```python
from build123d import *

# Parameters (mm, degrees)
SKETCH_1_R          = 3
EXTRUDE_1_DEPTH     = 4
SKETCH_2_W          = 102
SKETCH_2_H          = 85
EXTRUDE_2_DEPTH     = 50
SKETCH_4_W          = 96
SKETCH_4_H          = 79
CUT_EXTRUDE_3_DEPTH = 50
FILLET_1_R          = 4
CUT_EXTRUDE_4_REACH = 124.172
SKETCH_5_R          = 10


with BuildPart() as part:
    # 草图1 → 凸台-拉伸1 (new body)
    with BuildSketch(Plane(origin=(0, 0, 0), x_dir=(1, 0, 0), z_dir=(0, 1, 0))):
        Polygon((51, -42.5), (51, 42.5), (32.560911085, 54.5), (-32.560911085, 54.5), (-51, 42.5), (-51, -42.5), (-32.560911085, -54.5), (32.560911085, -54.5), align=None)
        with Locations(Location((-24, 48.5, 0), (0, 0, 270))):
            Circle(SKETCH_1_R, mode=Mode.SUBTRACT)
        with Locations(Location((24, 48.5, 0), (0, 0, 270))):
            Circle(SKETCH_1_R, mode=Mode.SUBTRACT)
        with Locations(Location((24, -48.5, 0), (0, 0, 270))):
            Circle(SKETCH_1_R, mode=Mode.SUBTRACT)
        with Locations(Location((-24, -48.5, 0), (0, 0, 270))):
            Circle(SKETCH_1_R, mode=Mode.SUBTRACT)
    extrude(amount=EXTRUDE_1_DEPTH)

    # 草图2 → 凸台-拉伸2 (add)
    with BuildSketch(Plane(origin=(0, 4, 0), x_dir=(1, 0, 0), z_dir=(0, 1, 0))):
        Rectangle(SKETCH_2_W, SKETCH_2_H)
    extrude(amount=EXTRUDE_2_DEPTH)

    # 草图4 → 切除-拉伸3 (cut)
    with BuildSketch(Plane.XZ):
        Rectangle(SKETCH_4_W, SKETCH_4_H)
    extrude(amount=-CUT_EXTRUDE_3_DEPTH, mode=Mode.SUBTRACT)

    # 圆角1
    fillet_1_edges = [part.edges().sort_by_distance(p)[0] for p in [
        (51, 54, 0),
        (0, 54, -42.5),
        (-51, 54, 0),
        (0, 54, 42.5),
    ]]
    fillet(fillet_1_edges, radius=FILLET_1_R)

    # 草图5 → 切除-拉伸4 (cut, up to next)
    with BuildSketch(Plane.XY.offset(42.5), mode=Mode.PRIVATE) as cut_extrude_4_sk1:
        with Locations((-31.111235747, 22.5989242)):
            Circle(SKETCH_5_R)
    cut_extrude_4_tool1 = extrude(cut_extrude_4_sk1.sketch, amount=-CUT_EXTRUDE_4_REACH, mode=Mode.PRIVATE) & part.part
    add(cut_extrude_4_tool1.solids().sort_by_distance((-31.111236, 22.598924, 42.5))[0], mode=Mode.SUBTRACT)


solid = part.part
```
CAD build for the part. Positions are in the model's coordinates, mm. A direction names the side the tool comes from. Round coordinates to 2 decimals unless told otherwise and drop trailing zeros. Write each loop counter-clockwise with the first axis right and the second up, starting at its lowest first coordinate (ties: lowest second). Pieces come first, ordered by that corner, then holes. Notation, with made-up numbers: M -25,-40 L -18,-40 A24 cw -18,-2 Z; hole C 45.25,79.5 d1. An arc over 180 degrees is marked long. One line per question, with ' | ' between items.
1. Pin check, flat tips, straight feed: pin 1 Ø12 at (x, y) = (-16.5, 15.5) entering from -Z; pin 2 Ø23 at (x, y) = (-31.11, 22.6) entering from +Z; pin 3 Ø13 at (x, z) = (19.5, -49.5) entering from +Y. Stop position of each tip, or through.
Working result:
pin 1: z = -42.5 | pin 2: z = 42.5 | pin 3: y = 4
2. Cut at C-C on y = 8. Write the cut outline in (x, z), and give its area (3 significant figures).
Working result:
outline: M -51,-42.5 L 51,-42.5 L 51,42.5 L -51,42.5 Z; hole M -48,-39.5 L 48,-39.5 L 48,39.5 L -48,39.5 Z | area: 1,090 mm2
3. Mould opens along X. For faces 4 (the flat face through (-1, 25, -39.5)), 5 (the flat face through (41.91, 1.972, -48.416)), 6 (the cylindrical face through (0.714, 52.797, 41.359)) say: pulls with the +X half, pulls with the -X half, needs draft (parallel to the pull), parting line crosses it, or undercut.
Working result:
face 4: undercut | face 5: pulls with the +X half | face 6: needs draft
4. Which spindle directions (+Z, -Z, +X, -X, +Y, -Y) get a long thin tool onto all of the face, cutting with end or side? Do faces 1 (the flat face through (-48, 25, -1)), 2 (the flat face through (-1, 27, -42.5)), 3 (the flat face through (-1, 4, 48)). Say none if no direction does.
Working result:
face 1: -Y | face 2: -Z, +X, -X, +Y | face 3: +Z, +X, -X, +Y
5. Cut at B-B on z = 48.5. Write the cut outline in (x, y).
Working result:
outline: M -41.78,0 L -27,0 L -27,4 L -41.78,4 Z; M -21,0 L 21,0 L 21,4 L -21,4 Z; M 27,0 L 41.78,0 L 41.78,4 L 27,4 Z
6. Cut at A-A on x = 24. Write the cut outline in (y, z), and give its area (3 significant figures).
Working result:
outline: M 0,-54.5 L 4,-54.5 L 4,-51.5 L 0,-51.5 Z; M 0,-45.5 L 4,-45.5 L 4,-42.5 L 50,-42.5 A4 ccw 54,-38.5 L 54,38.5 A4 ccw 50,42.5 L 4,42.5 L 4,45.5 L 0,45.5 L 0,39.5 L 50,39.5 L 50,-39.5 L 0,-39.5 Z; M 0,51.5 L 4,51.5 L 4,54.5 L 0,54.5 Z | area: 681 mm2
7. Probe L1, parallel to X at y = 22, z = -31; L2, parallel to Z at x = -9, y = 40; L3, parallel to X at y = 1, z = -48. List the from-to ranges inside material, lowest first. Write a range as from..to.
Working result:
L1: -51..-48, 48..51 | L2: -42.5..-39.5, 39.5..42.5 | L3: -42.55..-26.96, -21.04..21.04, 26.96..42.55
8. Cut at D-D on x = -24. Write the cut outline in (y, z), and give its area (3 significant figures).
Working result:
outline: M 0,-54.5 L 4,-54.5 L 4,-51.5 L 0,-51.5 Z; M 0,-45.5 L 4,-45.5 L 4,-42.5 L 50,-42.5 A4 ccw 54,-38.5 L 54,38.5 A4 ccw 50,42.5 L 29.63,42.5 L 29.63,39.5 L 50,39.5 L 50,-39.5 L 0,-39.5 Z; M 0,39.5 L 15.57,39.5 L 15.57,42.5 L 4,42.5 L 4,45.5 L 0,45.5 Z; M 0,51.5 L 4,51.5 L 4,54.5 L 0,54.5 Z | area: 639 mm2
